Here's how the part is built. I have some questions about the finished solid (model axes, mm). A direction names the side the tool comes from. Round coordinates to 2 decimals unless told otherwise and drop trailing zeros. Loops run counter-clockwise (first coordinate to the right, second up) from the corner with the lowest first, then second, coordinate; pieces in that order, holes last. Notation, with made-up numbers: M -31.5,24.25 L 6.5,24.25 A23 ccw 6.5,63.25 Z; hole C 65.5,-17 d3. An arc over 180 degrees is marked long. One line per question, with ' | ' between items. Start each with the question number.
```python
from build123d import *

# Parameters (mm, degrees)
SKETCH3_W           = 232.55
SKETCH3_H           = 63.5
SKETCH3_R           = 3.25
SKETCH3_R_2         = 2.778125
BOSS_EXTRUDE1_DEPTH = 10
CIRPATTERN1_COUNT   = 7
FILLET1_R           = 63.5
SKETCH5_R           = 3.25
CUT_EXTRUDE4_DEPTH  = 11


with BuildPart() as part:
    # Sketch3 → Boss-Extrude1 (new body)
    with BuildSketch(Plane(origin=(0, 0, 0), x_dir=(1, 0, 0), z_dir=(0, 1, 0))):
        with Locations((116.275, 0)):
            Rectangle(SKETCH3_W, SKETCH3_H)
        with Locations((200.8, 0)):
            Circle(SKETCH3_R, mode=Mode.SUBTRACT)
        with Locations((159.525, 22.225)):
            Circle(SKETCH3_R_2, mode=Mode.SUBTRACT)
        with Locations((159.525, -22.225)):
            Circle(SKETCH3_R_2, mode=Mode.SUBTRACT)
    boss_extrude1 = extrude(amount=BOSS_EXTRUDE1_DEPTH)

    # CirPattern1: Boss-Extrude1 ×7 about axis
    cirpattern1_axis = Axis((0, 0, 0), (0, 1, 0))
    for i in range(1, CIRPATTERN1_COUNT):
        add(boss_extrude1.rotate(cirpattern1_axis, i * 360 / CIRPATTERN1_COUNT))

    # Fillet1
    fillet1_edges = [part.edges().sort_by_distance(p)[0] for p in [
        (65.929554341, 5, 31.75),
        (65.929554341, 5, -31.75),
        (16.283255204, 5, 71.341602418),
        (-45.624667219, 5, 57.211523112),
        (-73.176284653, 5, 0),
        (-45.624667219, 5, -57.211523112),
        (16.283255204, 5, -71.341602418),
    ]]
    fillet(fillet1_edges, radius=FILLET1_R)

    # Sketch5 → Cut-Extrude4 (cut, through all)
    with BuildSketch(Plane(origin=(0, 0, 0), x_dir=(1, 0, 0), z_dir=(0, 1, 0))):
        with Locations((-75, 75)):
            Circle(SKETCH5_R)
        with Locations((75, 75)):
            Circle(SKETCH5_R)
        with Locations((75, -75)):
            Circle(SKETCH5_R)
        with Locations((-75, -75)):
            Circle(SKETCH5_R)
        Circle(SKETCH5_R)
    extrude(amount=CUT_EXTRUDE4_DEPTH, mode=Mode.SUBTRACT)


solid = part.part
```
1) Imagine slicing it at B-B (y = 1.75). State how many separate pieces and enclosed holes the cut face has, then the cut area to 3 significant figures.
2) Please list where these lines run through material, in increasing order: L1, parallel to X at y = 5.75, z = 0; L2, parallel to X at y = 4.75, z = -75; L3, parallel to Z at x = 200.8, y = 4.25. Write a range as from..to.
3) Imagine slicing it at A-A (x = -142.5). Write out the boundary of the cut face in (y, z), then the cut area to 3 significant figures.
4) We'd pull the mould along X, two halves only. Please class faces 1 (the face through (232.55, 5, 0)), 2 (the face through (-98.07, 5.07, -121.37)), 3 (the face through (-78.78, 4.93, -202.47)): pulls with the +X half, pulls with the -X half, needs draft (parallel to the pull), parting line crosses it, or undercut.
5) I'm going to push flat-ended pins straight in: pin 1 Ø4 at (y, z) = (6.5, -65) entering from +X; pin 2 Ø1 at (y, z) = (8.5, -139.5) entering from +X; pin 3 Ø5 at (x, z) = (-153.37, 49.19) entering from -Y; pin 4 Ø6 at (y, z) = (6.5, 136) entering from +X. Where does each tip first touch, or does it pass through?
6) For faces 4 (the face through (140.15, 4.93, 68.6)), 5 (the face through (-207.42, 4.93, 64.65)), 6 (the face through (215, 5, -31.75)), 7 (the face through (-179.87, 4.93, 121.86)), 8 (the face through (-179.87, 4.93, -121.86)), which set-ups out of +Z, -Z, +X, -X, +Y, -Y let a thin tool reach every point of the face, with its end or its side?
7) Imagine slicing it at C-C (z = 41). Write out the boundary of the cut face in (x, y), then the cut area to 3 significant figures.
Results are:
1) separate pieces: 1 | enclosed holes: 26 | area: 115,000 mm²
2) L1: -156.03..-3.25, 3.25..197.55, 204.05..232.55 | L2: -221.99..-78.25, -71.75..71.75, 78.25..137.6 | L3: -31.75..-3.25, 3.25..31.75
3) outline: M 0,-108.38 L 10,-108.38 L 10,108.38 L 0,108.38 Z | area: 2,170 mm²
4) face 1: pulls with the +X half | face 2: undercut | face 3: pulls with the -X half
5) pin 1: x = 143.09 | pin 2: x = 152.26 | pin 3: through | pin 4: x = 151.46
6) face 4: +X, +Y, -Y | face 5: -X, +Y, -Y | face 6: -Z, +X, +Y, -Y | face 7: +Z, +Y, -Y | face 8: -Z, +Y, -Y
7) outline: M -171.04,0 L 164.79,0 L 164.79,10 L -171.04,10 Z | area: 3,360 mm²
